Could you check a few things on this model? Use its own coordinates, in mm. Face numbers are marked on the shaded views. A direction names the side the tool comes from. Round coordinates to 2 decimals unless told otherwise and drop trailing zeros. Loops run counter-clockwise (first coordinate to the right, second up) from the corner with the lowest first, then second, coordinate; pieces in that order, holes last. Notation, with made-up numbers: (62, -9.5) -> (106, -9.5) arc R28 ccw to (106, 27.5) -> close; hole circle Ø8 at (72, -22.75). An arc over 180 degrees is marked (long way). Write each question's results on one line, items separated by ' | '.
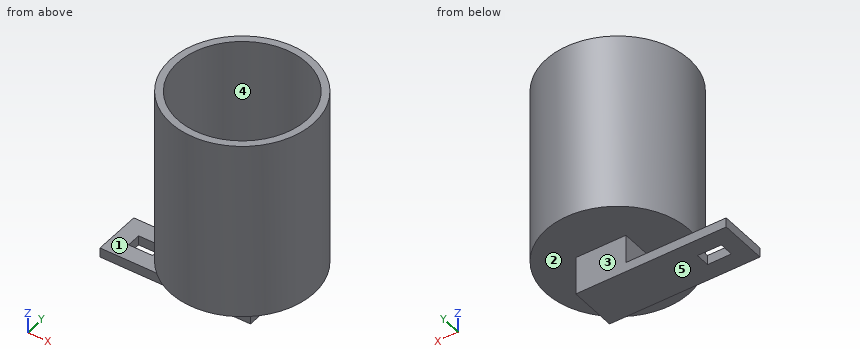
from build123d import *

# Parameters (mm, degrees)
ESQUISSE1_R             = 30
BOSS_EXTRU_1_DEPTH      = 75
ESQUISSE2_R             = 27
ENL_V_MAT_EXTRU_1_DEPTH = 70
ESQUISSE3_W             = 21
ESQUISSE3_H             = 20
BOSS_EXTRU_2_DEPTH      = 16
ESQUISSE4_W             = 4
ESQUISSE4_H             = 20
BOSS_EXTRU_3_DEPTH      = 42
ENL_V_MAT_EXTRU_2_REACH = 111.258
ESQUISSE5_W             = 10
ESQUISSE5_H             = 6


with BuildPart() as part:
    # Esquisse1 → Boss.-Extru.1 (new body)
    with BuildSketch(Plane.XY):
        Circle(ESQUISSE1_R)
    extrude(amount=BOSS_EXTRU_1_DEPTH)

    # Esquisse2 → Enlèv. mat.-Extru.1 (cut)
    with BuildSketch(Plane.XY.offset(75)):
        Circle(ESQUISSE2_R)
    extrude(amount=-ENL_V_MAT_EXTRU_1_DEPTH, mode=Mode.SUBTRACT)

    # Esquisse3 → Boss.-Extru.2 (add)
    with BuildSketch(Plane(origin=(0, 0, 0), x_dir=(-1, 0, 0), z_dir=(0, 0, -1))):
        Rectangle(ESQUISSE3_W, ESQUISSE3_H)
    extrude(amount=BOSS_EXTRU_2_DEPTH)

    # Esquisse4 → Boss.-Extru.3 (add)
    with BuildSketch(Plane.ZY.offset(10.5)):
        with Locations((-14, 0)):
            Rectangle(ESQUISSE4_W, ESQUISSE4_H)
    extrude(amount=BOSS_EXTRU_3_DEPTH)

    # Esquisse5 → Enlèv. mat.-Extru.2 (cut, up to next)
    with BuildSketch(Plane(origin=(0, 0, -16), x_dir=(-1, 0, 0), z_dir=(0, 0, -1)), mode=Mode.PRIVATE) as enl_v_mat_extru_2_sk1:
        with Locations((40.5, 0)):
            Rectangle(ESQUISSE5_W, ESQUISSE5_H)
    enl_v_mat_extru_2_tool1 = extrude(enl_v_mat_extru_2_sk1.sketch, amount=-ENL_V_MAT_EXTRU_2_REACH, mode=Mode.PRIVATE) & part.part
    add(enl_v_mat_extru_2_tool1.solids().sort_by_distance((-40.5, 0, -16))[0], mode=Mode.SUBTRACT)


solid = part.part
1) I want a section at C-C, the plane x = 0. Write out the boundary of the cut face in (y, z).
Model answer:
outline: (-30, 0) -> (-10, 0) -> (-10, -16) -> (10, -16) -> (10, 0) -> (30, 0) -> (30, 75) -> (27, 75) -> (27, 5) -> (-27, 5) -> (-27, 75) -> (-30, 75) -> close
2) I'm going to push flat-ended pins straight in: pin 1 (3.5 mm diameter, centred on y = 3, z = -7, fed in from -X); pin 2 (8 mm diameter, centred on x = -23, z = -4.5, fed in from +Y); pin 3 (3 mm diameter, centred on x = 17.5, y = -22.5, fed in from -Z); pin 4 (4.5 mm diameter, centred on x = -42.5, z = -13, fed in from +Y). Where does each tip first touch, or does it pass through?
Model answer:
pin 1: stops at x = -10.5 | pin 2: passes through | pin 3: stops at z = 0 | pin 4: stops at y = 10
3) I want a section at A-A, the plane x = -42. Write out the boundary of the cut face in (y, z).
Model answer:
outline: (-10, -16) -> (-3, -16) -> (-3, -12) -> (-10, -12) -> close; (3, -16) -> (10, -16) -> (10, -12) -> (3, -12) -> close
4) For the marked faces 1 and 2, which set-ups out of +Z, -Z, +X, -X, +Y, -Y let a thin tool reach every point of the face, with its end or its side?
Model answer:
face 1: -X, +Y, -Y | face 2: none
5) If we mould it in two halves opening along Y, with no side actions, what happens to the marked faces 3, 4 and 5? For each: released by +Y, released by -Y, zero draft, split by the parting line, or undercut.
Model answer:
face 3: released by +Y | face 4: undercut | face 5: zero draft
6) I want a section at B-B, the plane y = 0. Write out the boundary of the cut face in (x, z).
Model answer:
outline: (-52.5, -16) -> (-45.5, -16) -> (-45.5, -12) -> (-52.5, -12) -> close; (-35.5, -16) -> (10.5, -16) -> (10.5, 0) -> (30, 0) -> (30, 75) -> (27, 75) -> (27, 5) -> (-27, 5) -> (-27, 75) -> (-30, 75) -> (-30, 0) -> (-10.5, 0) -> (-10.5, -12) -> (-35.5, -12) -> close
7) I want a section at D-D, the plane z = 26.5. Write out the boundary of the cut face in (x, y), plus the area to 3 significant figures.
Model answer:
outline: circle Ø60 at (0, 0); hole circle Ø54 at (0, 0) | area: 537 mm2
8) I need wall thicknesses on line 1 (Y direction, x = 0, z = 25.5); line 2 (Z direction, x = -19, y = 9); line 3 (X direction, y = -5, z = 69). Which ranges of each line are inside material? Lowest first, please.
Model answer:
line 1: y = -30 to -27, 27 to 30 | line 2: z = -16 to -12, 0 to 5 | line 3: x = -29.58 to -26.53, 26.53 to 29.58
